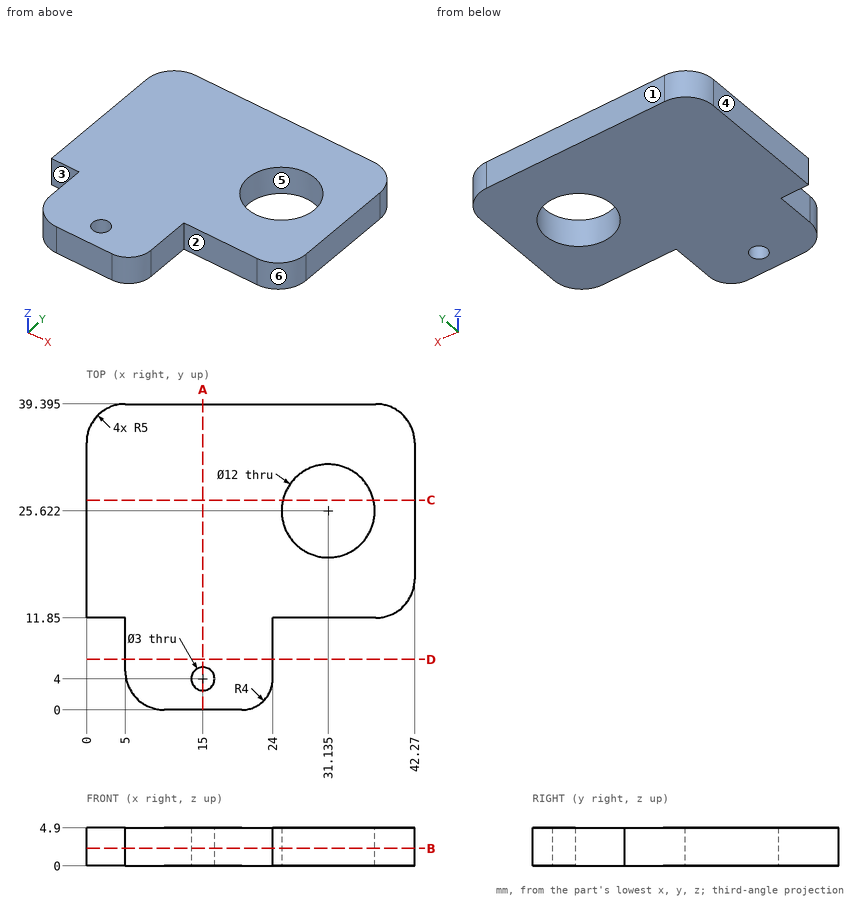
For this review, use the dimensioned drawing (mm, ordinates from the lowest corner) and the shaded views. A direction names the side the tool comes from. Coordinates: 2 decimals unless noted, no trailing zeros. Write each loop counter-clockwise with the first axis right and the second up, starting at its lowest first coordinate (ties: lowest second). Pieces come first, ordered by that corner, then holes. Notation, with made-up numbers: (-38, 82.25) - (19, 82.25) arc R4 ccw to (19, 88.25) - close; hole circle Ø7 at (62, -4.5). An arc over 180 degrees is marked (long way). One line per item, written item: value.
1) Add section B-B (z = 2.25). Give the number of separate pieces and of enclosed holes in the cut face, plus the area to 3 significant figures.
Answer sheet:
separate pieces: 1
enclosed holes: 2
area: 1,240 mm2
2) Add section A-A (x = 15). State the section outline as (y, z) points (1 decimal), plus the area to 3 significant figures.
Answer sheet:
outline: (0, 0) - (2.5, 0) - (2.5, 4.9) - (0, 4.9) - close; (5.5, 0) - (39.4, 0) - (39.4, 4.9) - (5.5, 4.9) - close
area: 178 mm2
3) Add section D-D (y = 6.5). State the section outline as (x, z) points.
Answer sheet:
outline: (5, 0) - (24, 0) - (24, 4.9) - (5, 4.9) - close
4) Add section C-C (y = 27). State the section outline as (x, z) points (1 decimal).
Answer sheet:
outline: (0, 0) - (25.3, 0) - (25.3, 4.9) - (0, 4.9) - close; (37, 0) - (42.3, 0) - (42.3, 4.9) - (37, 4.9) - close
5) For the marked faces 1, 2 and 3, list the 3-axis set-ups (+Z, -Z, +X, -X, +Y, -Y) from which the entire face can be reached by the end or side of a thin tool; tool diameter is ignored.
Answer sheet:
face 1: +Z, -Z, +X, -X, +Y
face 2: +Z, -Z, +X, -Y
face 3: +Z, -Z, -X, -Y
6) Insertion check: pin 1 (3 mm diameter, centred on x = 19, y = 20.5, fed in from -Z). The pin has a flat end and moves straight along its axis. Give the tip position at first contact, or say it passes through.
Answer sheet:
pin 1: stops at z = 0
7) Mouldability with a two-part tool opening along Y and no side actions: class the marked faces 4, 5 and 6 as +Y half, -Y half, draft (parallel to the pull), parting line (faces both ways), or undercut.
Answer sheet:
face 4: draft
face 5: undercut
face 6: -Y half
8) To check wall thickness, follow probe 1 along Y at (x, z) = (15, 1.7) (1 decimal); probe 2 along X at (y, z) = (6, 1.6); probe 3 along X at (y, z) = (20.5, 0.75). State the ranges of each line that lie inside material, in increasing order.
Answer sheet:
probe 1: y = 0 to 2.5, 5.5 to 39.4
probe 2: x = 5 to 24
probe 3: x = 0 to 28.01, 34.26 to 42.27
